Geometry check sheet. Reference: the model listing, model coordinates, mm. A direction names the side the tool comes from. Round coordinates to 2 decimals unless told otherwise and drop trailing zeros. Write each loop counter-clockwise with the first axis right and the second up, starting at its lowest first coordinate (ties: lowest second). Pieces come first, ordered by that corner, then holes.
Item 1: Draft check along X on faces 6 (the face through (-31, 0, -6)), 7 (the face through (-1, 0, -32)), 8 (the face through (100, -2, -16)). Enter one of: pulls with the +X half, pulls with the -X half, needs draft (parallel to the pull), parting line crosses it, or undercut.
Item 2: Cross-section at A-A (z = -3). Enter the section's corners in (x, y), then the cut area to 3 significant figures.
Item 3: Scan lines: probe 1 along X at (y, z) = (-7.75, -20); probe 2 along Y at (x, z) = (89, -21); probe 3 along Z at (x, y) = (-27, 1). Record each from-to range of solid material in increasing order.
Item 4: Cross-section at B-B (z = -19). Enter the section's corners in (x, y).
Item 5: Depth check by flat-ended pin: P1, Ø0.8, axis at y = -0.5, z = -9, coming from the +X side; P2, Ø3, axis at x = -86.5, z = -9, coming from the -Y side; P3, Ø0.8, axis at x = 85.5, y = 0, coming from the +Z side. Enter the tip coordinate at first touch or a pass-through.
Item 6: Access from +Z, -Z, +X, -X, +Y, -Y to the whole of each face (thin tool, end or side, straight path). Record for faces 1 (the face through (90, 1.25, -11)), 2 (the face through (-85, -7, -11)), 3 (the face through (-1, 9, -16)), 4 (the face through (-85, 7, -11)), 5 (the face through (-42, 0, -3)).
from build123d import *

# Parameters (mm, degrees)
SKETCH002_W  = 200
SKETCH002_H  = 18
PAD001_DEPTH = 10
PAD_DEPTH    = 22
SKETCH001_W  = 22
SKETCH001_H  = 8
POCKET_DEPTH = 6


with BuildPart() as base:
    # Sketch002 → Pad001 (new body)
    with BuildSketch(Plane.XY):
        Rectangle(SKETCH002_W, SKETCH002_H)
    extrude(amount=PAD001_DEPTH)


with BuildPart() as base_1:
    # Body001 placement: moved
    add(base.part.moved(Location((0, 0, -32))))


with BuildPart() as model_fusion:
    # Sketch → Pad (new body)
    with BuildSketch(Plane.XY):
        Polygon((-100, 9), (-90, 9), (-90, 7), (-80, 7), (-80, 9), (100, 9), (100, 1.25), (79, 1.25), (79, -1.25), (100, -1.25), (100, -9), (-80, -9), (-80, -7), (-90, -7), (-90, -9), (-100, -9), align=None)
    extrude(amount=PAD_DEPTH)

    # Sketch001 (on Face18 of Pad) → Pocket (cut)
    with BuildSketch(Plane.XY.offset(22)):
        with Locations((-31, 0)):
            Rectangle(SKETCH001_W, SKETCH001_H)
    extrude(amount=-POCKET_DEPTH, mode=Mode.SUBTRACT)


with BuildPart() as model_fusion_1:
    # Body placement: moved
    add(model_fusion.part.moved(Location((0, 0, -22))))

    # Fusion: union Base
    add(base_1.part)


solid = model_fusion_1.part
Resolved:
1. face 6: undercut
1. face 7: needs draft
1. face 8: pulls with the +X half
2. outline: (-100, -9) - (-90, -9) - (-90, -7) - (-80, -7) - (-80, -9) - (100, -9) - (100, -1.25) - (79, -1.25) - (79, 1.25) - (100, 1.25) - (100, 9) - (-80, 9) - (-80, 7) - (-90, 7) - (-90, 9) - (-100, 9) - close; hole (-42, -4) - (-20, -4) - (-20, 4) - (-42, 4) - close
2. area: 3,330 mm2
3. probe 1: x = -100 to -90, -80 to 100
3. probe 2: y = -9 to -1.25, 1.25 to 9
3. probe 3: z = -32 to -6
4. outline: (-100, -9) - (-90, -9) - (-90, -7) - (-80, -7) - (-80, -9) - (100, -9) - (100, -1.25) - (79, -1.25) - (79, 1.25) - (100, 1.25) - (100, 9) - (-80, 9) - (-80, 7) - (-90, 7) - (-90, 9) - (-100, 9) - close
5. P1: stops at x = 79
5. P2: stops at y = -7
5. P3: stops at z = -22
6. face 1: +Z, +X
6. face 2: +Z, -Y
6. face 3: +Z, -Z, +X, -X, +Y
6. face 4: +Z, +Y
6. face 5: +Z
